Autodesk Inventor part; units mm, degrees
ref_plane "YZ Plane" through (0, 0, 0) normal (1, 0, 0) x (0, 1, 0)
ref_plane "XZ Plane" through (0, 0, 0) normal (0, 1, 0) x (-1, 0, 0)
ref_plane "XY Plane" through (0, 0, 0) normal (0, 0, 1) x (1, 0, 0)
sketch "Sketch1" plane through (0, 0, 0) normal (0, 1, 0) x (-1, 0, 0)
  circle A0 centre (0, 0) radius 18.925
  circle A1 centre (0, 0) radius 8.925
  dimension "d0" = 37.85
  dimension "d1" = 17.85
extrude "Extrusion1" add sketch "Sketch1" along normal blind 2
sketch "Sketch2" plane through (0, 2, 0) normal (0, 1, 0) x (1, 0, 0)
  line L0 (-23.925, -1) -> (-13.925, -1)
  line L1 (-13.925, -1) -> (-13.925, 1)
  line L2 (-13.925, 1) -> (-23.925, 1)
  line L3 (-23.925, 1) -> (-23.925, -1)
  point P0 (0, 0)
  dimension "d4" = 1
  dimension "d5" = 2
  dimension "d6" = 13.925
  dimension "d7" = 10
extrude "Extrusion2" cut sketch "Sketch2" against normal blind 2
pattern_circular "Circular Pattern1" count 6 over 360 about axis through (0, -10, 0) along (0, 1, 0) of "Extrusion2"
sketch "Sketch3" plane through (0, 2, 0) normal (0, 1, 0) x (1, 0, 0)
  circle A0 centre (-7.7293, -4.4625) radius 3.5
  line L0 (-7.7293, -4.4625) -> (0, 0) construction
  circle A1 centre (0, 0) radius 8.925
  line L1 (-26.458, 0) -> (26.458, 0)
  dimension "d13" = 30
  dimension "d14" = 7
extrude "Extrusion3" cut sketch "Sketch3" against normal blind 2 contours A0 A1 | A1 A0
pattern_circular "Circular Pattern2" count 6 over 360 about axis through (0, -10, 0) along (0, 1, 0) of "Extrusion3"
properties part number "Ring_n6"
Part model, mm, in its own coordinate system. A direction names the side the tool comes from. Coordinates: 2 decimals unless noted, no trailing zeros. Order: outer loops, then holes, each group sorted by start corner. A loop starts at its lowest first (then second) coordinate and runs counter-clockwise, first axis right, second up. Notation, with made-up numbers: M 47,61.25 L 56,61.25 A37 cw 56,100.25 Z; hole C -8.75,55 d11. An arc over 180 degrees is marked long. Use a Markdown table: item, result.
(1) Flat gauge pins, fed straight in: pin 1 (3 mm diameter, centred on x = 13, z = -12, fed in from -Y); pin 2 (5.5 mm diameter, centred on x = 7.73, z = -4.46, fed in from -Y); pin 3 (0.6 mm diameter, centred on x = -16, y = 1.5, fed in from +Z); pin 4 (1 mm diameter, centred on y = 1.5, z = -3, fed in from +X). Where does each tip first touch, or does it go through?
A:
| item | result |
|---|---|
| pin 1 | stops at y = 0 |
| pin 2 | passes through |
| pin 3 | stops at z = 10.57 |
| pin 4 | stops at x = 18.76 |
(2) Tool access for faces 4 (the cylindrical face through (-16.327, 0.986, 9.57)), 5 (the flat face through (16, 1, 1)), 6 (the cylindrical face through (-4.449, 0.986, 7.737)): list every direction of +Z, -Z, +X, -X, +Y, -Y with a clear straight run to the whole face (end or side of a thin tool).
A:
| item | result |
|---|---|
| face 4 | +Z, -X, +Y, -Y |
| face 5 | +X, +Y, -Y |
| face 6 | +Y, -Y |
(3) Cut at B-B on z = 14. Write the cut outline in (x, y).
A:
| item | result |
|---|---|
| outline | M -12.73,0 L -9.24,0 L -9.24,2 L -12.73,2 Z; M -6.93,0 L 6.93,0 L 6.93,2 L -6.93,2 Z; M 9.24,0 L 12.73,0 L 12.73,2 L 9.24,2 Z |
(4) Pull direction Z, two halves, no side cores. Call faces 1 (the cylindrical face through (16.452, 0.986, 9.354)), 2 (the cylindrical face through (16.327, 0.986, -9.57)), 3 (the flat face through (-16, 1, 1)): released by +Z, released by -Z, zero draft, split by the parting line, or undercut.
A:
| item | result |
|---|---|
| face 1 | released by +Z |
| face 2 | released by -Z |
| face 3 | undercut |
(5) Cut at C-C on z = 9. Write the cut outline in (x, y).
A:
| item | result |
|---|---|
| outline | M -16.65,0 L -3.5,0 L -3.5,2 L -16.65,2 Z; M 3.5,0 L 16.65,0 L 16.65,2 L 3.5,2 Z |
(6) Probe L1, parallel to Z at x = 8.5, y = 0.5; L2, parallel to Z at x = -9.5, y = 0.5; L3, parallel to X at y = 1.15, z = 12. List the from-to ranges inside material, lowest first.
A:
| item | result |
|---|---|
| L1 | z = -16.91 to -16.72, -12.72 to -7.88, 7.88 to 12.72, 16.72 to 16.91 |
| L2 | z = -14.45 to -7.48, -1.44 to 1.44, 7.48 to 14.45 |
| L3 | x = -14.63 to -8.08, -7.07 to -1.67, 1.67 to 7.07, 8.08 to 14.63 |
(7) Cut at A-A on x = 2.5. Write the cut outline in (y, z), then the cut area to 3 significant figures.
A:
| item | result |
|---|---|
| outline | M 0,-18.76 L 2,-18.76 L 2,-11.37 L 0,-11.37 Z; M 0,11.37 L 2,11.37 L 2,18.76 L 0,18.76 Z |
| area | 29.5 mm^2 |
